For this review, use the dimensioned drawing (mm, ordinates from the lowest corner) and the shaded views. Give positions to 0.01 mm unless a question says otherwise; leave off trailing zeros. Loops run counter-clockwise (first coordinate to the right, second up) from the corner with the lowest first, then second, coordinate; pieces in that order, holes last. Notation, with made-up numbers: (-8, -13) -> (42, -13) arc R35 ccw to (42, 25) -> close; hole circle Ø1 at (56, 61). An arc over 180 degrees is marked (long way). Write each question's results on one line, items separated by ' | '. Start each with the question number.
Q1. Mouldability with a two-part tool opening along Y and no side actions: class the marked faces 1, 2, 3 and 4 as released by +Y, released by -Y, zero draft, split by the parting line, or undercut.
Q2. We need section C-C (y = 5). Write out the cut boundary in (x, z), plus the area to 3 significant figures.
Q3. We need section D-D (z = 8.5). Write out the cut boundary in (x, y).
Q4. We need section B-B (z = 5). Write out the cut boundary in (x, y).
Q5. We need section A-A (x = 12.5). Write out the cut boundary in (y, z).
Q6. Wall thickness on L1, parallel to Y at x = 20, z = 4.25; L2, parallel to X at y = 2.5, z = 5; L3, parallel to X at y = 4.75, z = 6.5: over which ranges is each line inside the solid? List them lowest first. Write a range as [from, to].
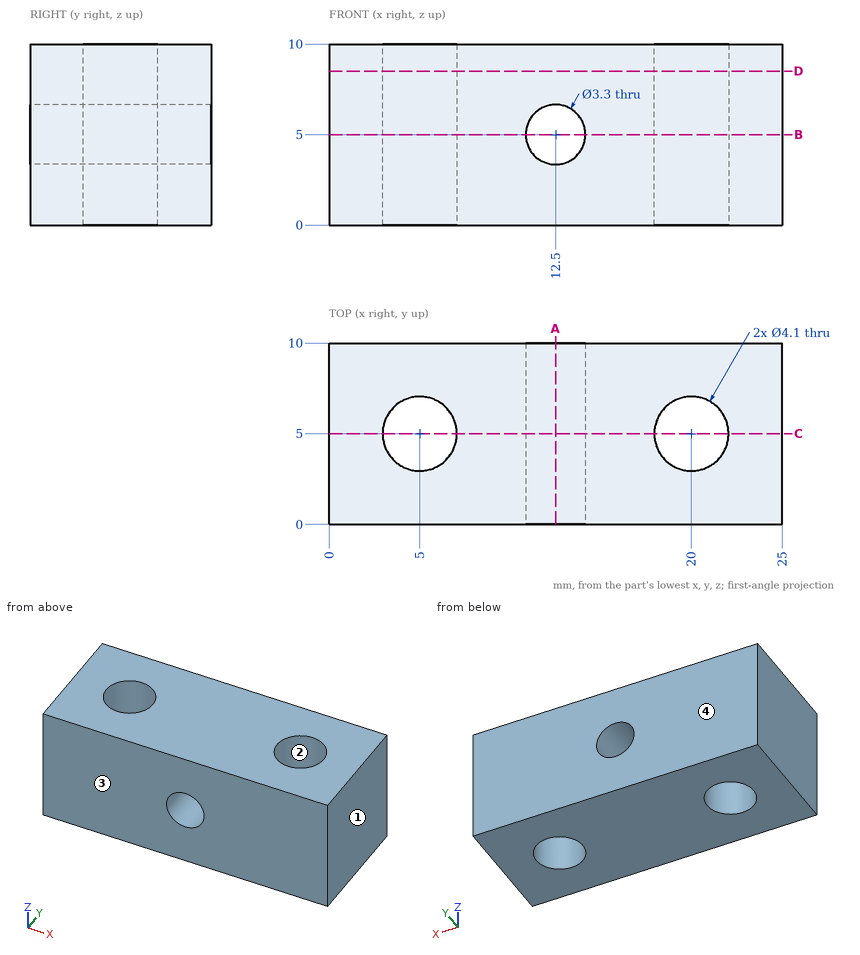
Output:
1) face 1: zero draft | face 2: undercut | face 3: released by -Y | face 4: released by +Y
2) outline: (0, 0) -> (2.95, 0) -> (2.95, 10) -> (0, 10) -> close; (7.05, 0) -> (17.95, 0) -> (17.95, 10) -> (7.05, 10) -> close; (22.05, 0) -> (25, 0) -> (25, 10) -> (22.05, 10) -> close; hole circle Ø3.3 at (12.5, 5) | area: 159 mm2
3) outline: (0, 0) -> (25, 0) -> (25, 10) -> (0, 10) -> close; hole circle Ø4.1 at (5, 5); hole circle Ø4.1 at (20, 5)
4) outline: (0, 0) -> (10.85, 0) -> (10.85, 10) -> (0, 10) -> close; (14.15, 0) -> (25, 0) -> (25, 10) -> (14.15, 10) -> close; hole circle Ø4.1 at (5, 5); hole circle Ø4.1 at (20, 5)
5) outline: (0, 0) -> (10, 0) -> (10, 3.35) -> (0, 3.35) -> close; (0, 6.65) -> (10, 6.65) -> (10, 10) -> (0, 10) -> close
6) L1: [0, 2.95], [7.05, 10] | L2: [0, 10.85], [14.15, 25] | L3: [0, 2.97], [7.03, 11.81], [13.19, 17.97], [22.03, 25]
